Geometry: final body of the model. Coordinates: model frame, mm. A direction names the side the tool comes from. Give positions to 0.01 mm unless a question says otherwise; leave off trailing zeros. Write each loop counter-clockwise with the first axis right and the second up, starting at its lowest first coordinate (ties: lowest second). Pieces come first, ordered by that corner, then holes. Notation, with made-up numbers: (22.25, 15) -> (35.25, 15) arc R33 cw to (35.25, 53) -> close; hole circle Ø9 at (2.25, -23). An arc over 180 degrees is marked (long way). Answer as a JSON object with one key per item and string values. Group by question number.
(1) Draft query along Y for faces 4 (the face through (5.058, 33, 11)), 5 (the face through (2.56, 29.78, 7.3)), 6 (the face through (27, 0, 6)). Return one class per face: +Y half, -Y half, draft (parallel to the pull), parting line (faces both ways), or undercut.
(2) Section query D-D on y = 31. Output: boundary loops of the cut face in (x, z) (3 decimals).
(3) Section query C-C on x = 26. Output: boundary loops of the cut face in (y, z) (3 decimals), plus the area to 3 significant figures.
(4) Contact query for a flat-ended pin moving along its axis: pin 1 Ø4 at (x, z) = (8, 4.5) entering from +Y. Output: stop coordinate, or through.
(5) Section query B-B on x = 50. Output: boundary loops of the cut face in (y, z) (1 decimal).
(6) Material intervals for probe 1 along X at (y, z) = (2, 7.75) (3 decimals); probe 2 along X at (y, z) = (37, 9.5) (3 decimals); probe 3 along Y at (x, z) = (10.5, 8), sorted ascending.
(7) Section query A-A on y = 5.5. Output: boundary loops of the cut face in (x, z) (3 decimals), plus the area to 3 significant figures.
(8) Set-up query: faces 1 (the face through (48.917, 33, 11)), 2 (the face through (3.086, 37.447, 15.727)), 3 (the face through (0.522, 36.519, 3.342)). Return all of +Z, -Z, +X, -X, +Y, -Y with unobstructed straight access to the full face (end or side cutting, diameter ignored); none if empty.
from build123d import *

# Parameters (mm, degrees)
BOSS_EXTRUDE1_DEPTH = 22.225
FILLET1_R           = 11.1125
CUT_EXTRUDE1_REACH  = 72.586
SKETCH4_R           = 4
SKETCH4_R_2         = 1
CIRPATTERN1_COUNT   = 4
SKETCH5_R           = 4
SKETCH5_R_2         = 1
CUT_EXTRUDE2_DEPTH  = 1.058333333
CIRPATTERN2_COUNT   = 4
SKETCH6_R           = 1
CUT_EXTRUDE3_DEPTH  = 1.058333333
BOSS_EXTRUDE2_START = 4
SKETCH7_R           = 10
SKETCH7_R_2         = 1
SKETCH7_R_3         = 4
BOSS_EXTRUDE2_DEPTH = 4


with BuildPart() as part:
    # Sketch2 → Boss-Extrude1 (new body)
    with BuildSketch(Plane.XY):
        Polygon((0, 39.6875), (0, 0), (53.975, 0), (53.975, 39.6875), (52.916666667, 39.6875), (52.916666667, 1.058333333), (1.058333333, 1.058333333), (1.058333333, 39.6875), align=None)
    extrude(amount=BOSS_EXTRUDE1_DEPTH)

    # Fillet1
    fillet1_edges = [part.edges().sort_by_distance(p)[0] for p in [
        (0.529166667, 39.6875, 0),
        (0.529166667, 39.6875, 22.225),
        (53.445833333, 39.6875, 0),
        (53.445833333, 39.6875, 22.225),
    ]]
    fillet(fillet1_edges, radius=FILLET1_R - 0.0001)  # a hair under: the kernel refuses the full size

    # Cut-Extrude1: up to this face of the body (flat: up to its plane)
    cut_extrude1_end = Plane(part.part.faces().sort_by_distance((0, 18.733844913, 11.1125))[0])
    # Sketch4 → Cut-Extrude1 (cut, up to the picked face)
    with BuildSketch(Plane(origin=(53.975, 0, 0), x_dir=(0, 0, -1), z_dir=(1, 0, 0)), mode=Mode.PRIVATE) as cut_extrude1_sk1:
        with Locations((-11.1125, 28.575)):
            Circle(SKETCH4_R)
    cut_extrude1_tool1 = split(extrude(cut_extrude1_sk1.sketch, amount=-CUT_EXTRUDE1_REACH, mode=Mode.PRIVATE), bisect_by=cut_extrude1_end, keep=Keep.BOTH, mode=Mode.PRIVATE)
    # Sketch4 → Cut-Extrude1 (cut, up to the picked face)
    with BuildSketch(Plane(origin=(53.975, 0, 0), x_dir=(0, 0, -1), z_dir=(1, 0, 0)), mode=Mode.PRIVATE) as cut_extrude1_sk2:
        with Locations((-11.1125, 35.575)):
            Circle(SKETCH4_R_2)
    cut_extrude1_tool2 = split(extrude(cut_extrude1_sk2.sketch, amount=-CUT_EXTRUDE1_REACH, mode=Mode.PRIVATE), bisect_by=cut_extrude1_end, keep=Keep.BOTH, mode=Mode.PRIVATE)
    cut_extrude1_1 = cut_extrude1_tool1.solids().sort_by(Axis((53.975, 28.575, 11.1125), (-1, 0, 0)))[0]
    add(cut_extrude1_1, mode=Mode.SUBTRACT)
    cut_extrude1_2 = cut_extrude1_tool2.solids().sort_by(Axis((53.975, 35.575, 11.1125), (-1, 0, 0)))[0]
    add(cut_extrude1_2, mode=Mode.SUBTRACT)
    cut_extrude1 = cut_extrude1_1 + cut_extrude1_2  # Cut-Extrude1 as one shape, for the pattern or mirror that repeats it

    # CirPattern1: Cut-Extrude1 ×4 about axis
    cirpattern1_axis = Axis((0, 28.575, 11.1125), (1, 0, 0))
    for i in range(1, CIRPATTERN1_COUNT):
        add(cut_extrude1.rotate(cirpattern1_axis, i * 360 / CIRPATTERN1_COUNT), mode=Mode.SUBTRACT)

    # Sketch5 → Cut-Extrude2 (cut)
    with BuildSketch(Plane.XZ):
        with Locations(Location((26.9875, 11.1125, 0), (0, 0, 270))):
            Circle(SKETCH5_R)
        with Locations(Location((22.037752532, 6.162752532, 0), (0, 0, 270))):
            Circle(SKETCH5_R_2)
    cut_extrude2 = extrude(amount=-CUT_EXTRUDE2_DEPTH, mode=Mode.SUBTRACT)

    # CirPattern2: Cut-Extrude2 ×4 about axis
    cirpattern2_axis = Axis((26.9875, 0, 11.1125), (0, 1, 0))
    for i in range(1, CIRPATTERN2_COUNT):
        add(cut_extrude2.rotate(cirpattern2_axis, i * 360 / CIRPATTERN2_COUNT), mode=Mode.SUBTRACT)

    # Sketch6 → Cut-Extrude3 (cut)
    with BuildSketch(Plane.XZ):
        with Locations(Location((13.4875, 11.1125, 0), (0, 0, 270))):
            Circle(SKETCH6_R)
        with Locations(Location((40.4875, 11.1125, 0), (0, 0, 270))):
            Circle(SKETCH6_R)
    extrude(amount=-CUT_EXTRUDE3_DEPTH, mode=Mode.SUBTRACT)

    # Sketch7 → Boss-Extrude2 (add)
    with BuildSketch(Plane(origin=(1.058333333, 0, 0), x_dir=(0, 0, -1), z_dir=(1, 0, 0)).offset(BOSS_EXTRUDE2_START)):
        with Locations(Location((-11.1125, 28.575, 0), (0, 0, 180))):
            Circle(SKETCH7_R)
        with Locations((-18.1125, 28.575)):
            Circle(SKETCH7_R_2, mode=Mode.SUBTRACT)
        with Locations((-11.1125, 21.575)):
            Circle(SKETCH7_R_2, mode=Mode.SUBTRACT)
        with Locations((-4.1125, 28.575)):
            Circle(SKETCH7_R_2, mode=Mode.SUBTRACT)
        with Locations((-11.1125, 35.575)):
            Circle(SKETCH7_R_2, mode=Mode.SUBTRACT)
        with Locations((-11.1125, 28.575)):
            Circle(SKETCH7_R_3, mode=Mode.SUBTRACT)
    boss_extrude2 = extrude(amount=-BOSS_EXTRUDE2_DEPTH)

    # Mirror1: Boss-Extrude2 across plane
    add(boss_extrude2.mirror(Plane.ZY.offset(-26.9875)))


solid = part.part
Answer list:
{
 "1": {"face 4": "draft", "face 5": "undercut", "face 6": "-Y half"},
 "2": {"outline": "(0, 0.268) -> (1.058, 0.268) -> (1.058, 1.411) -> (5.058, 1.411) -> (5.058, 7.931) -> (0, 7.931) -> close; (0, 14.294) -> (5.058, 14.294) -> (5.058, 20.814) -> (1.058, 20.814) -> (1.058, 21.957) -> (0, 21.957) -> close; (48.917, 1.411) -> (52.917, 1.411) -> (52.917, 0.268) -> (53.975, 0.268) -> (53.975, 7.931) -> (48.917, 7.931) -> close; (48.917, 14.294) -> (53.975, 14.294) -> (53.975, 21.957) -> (52.917, 21.957) -> (52.917, 20.814) -> (48.917, 20.814) -> close"},
 "3": {"outline": "(0, 0) -> (1.058, 0) -> (1.058, 7.236) -> (0, 7.236) -> close; (0, 14.989) -> (1.058, 14.989) -> (1.058, 22.225) -> (0, 22.225) -> close", "area": "15.3 mm2"},
 "4": {"pin 1": "y = 1.06"},
 "5": {"outline": "(0, 0) -> (1.1, 0) -> (1.1, 22.2) -> (0, 22.2) -> close; circle Ø20 at (28.6, 11.1); hole circle Ø2 at (21.6, 11.1); hole circle Ø8 at (28.6, 11.1); hole circle Ø2 at (28.6, 4.1); hole circle Ø2 at (28.6, 18.1); hole circle Ø2 at (35.6, 11.1)"},
 "6": {"probe 1": "0 to 1.058, 52.917 to 53.975", "probe 2": "0 to 5.058, 48.917 to 53.975", "probe 3": "0 to 1.06"},
 "7": {"outline": "(0, 0) -> (1.058, 0) -> (1.058, 22.225) -> (0, 22.225) -> close; (52.917, 0) -> (53.975, 0) -> (53.975, 22.225) -> (52.917, 22.225) -> close", "area": "47.0 mm2"},
 "8": {"face 1": "+Z, -Z, +Y", "face 2": "none", "face 3": "-Z, +X, -X, +Y"}
}
